Autodesk Inventor part; units mm, degrees
ref_plane "工作平面1" through (0, 5, 0) normal (0, -1, 0) x (1, 0, 0)
ref_plane "YZ Plane" through (0, 0, 0) normal (1, 0, 0) x (0, 1, 0)
ref_plane "XZ Plane" through (0, 0, 0) normal (0, 1, 0) x (-1, 0, 0)
sketch "草圖1" plane through (0, 0, 0) normal (0, 1, 0) x (-1, 0, 0)
  circle A0 centre (0, 0) radius 2.45
  dimension "d0" = 4.9
extrude "擠出1" add sketch "草圖1" along normal blind 160
ref_plane "工作平面1" through (0, 5, 0) normal (0, -1, 0) x (1, 0, 0)
sketch "草圖3" plane through (0, 5, 0) normal (0, -1, 0) x (1, 0, 0)
  circle A0 centre (0, 0) radius 2.45
  circle A1 centre (0, 0) radius 3.25
  line L0 (3.25, 0) -> (-3.25, 0)
  line L1 (-3.25, 0) -> (-3.25, -12)
  line L2 (-3.25, -12) -> (3.25, -12)
  line L3 (3.25, -12) -> (3.25, 0)
  line L4 (1.6, -12) -> (-1.6, -12)
  line L5 (-1.6, -12) -> (-1.6, -7)
  line L6 (-1.6, -7) -> (1.6, -7)
  line L7 (1.6, -7) -> (1.6, -12)
  line L8 (1.55, -7) -> (-1.55, -7)
  line L9 (-1.55, -7) -> (-1.55, -10.1)
  line L10 (-1.55, -10.1) -> (1.55, -10.1)
  line L11 (1.55, -10.1) -> (1.55, -7)
  line L12 (1.55, -10.1) -> (1.35, -10.1)
  line L13 (1.35, -10.1) -> (1.6, -12)
  line L14 (-1.55, -10.1) -> (-1.35, -10.1)
  line L15 (-1.35, -10.1) -> (-1.6, -12)
  circle A2 centre (0, -8.55) radius 2.192
  line L16 (-3.25, 0) -> (-3.25, 12)
  line L17 (-3.25, 12) -> (3.25, 12)
  line L18 (3.25, 12) -> (3.25, 0)
  line L19 (1.6, 12) -> (-1.6, 12)
  line L20 (-1.6, 12) -> (-1.6, 7)
  line L21 (-1.6, 7) -> (1.6, 7)
  line L22 (1.6, 7) -> (1.6, 12)
  line L23 (1.55, 7) -> (-1.55, 7)
  line L24 (-1.55, 7) -> (-1.55, 10.1)
  line L25 (-1.55, 10.1) -> (1.55, 10.1)
  line L26 (1.55, 10.1) -> (1.55, 7)
  line L27 (1.55, 10.1) -> (1.35, 10.1)
  line L28 (1.35, 10.1) -> (1.6, 12)
  line L29 (-1.55, 10.1) -> (-1.35, 10.1)
  line L30 (-1.35, 10.1) -> (-1.6, 12)
  circle A3 centre (0, 8.55) radius 2.192
  point P0 (0, -12)
  point P1 (0, -12)
  point P2 (0, -7)
  point P3 (-1.55, -7)
  point P4 (1.55, -7)
  point P5 (-1.55, -8.55)
  point P6 (-1.3711, -10.2603)
  point P7 (1.3711, -10.2603)
  point P8 (0, 12)
  point P9 (0, 12)
  point P10 (0, 7)
  point P11 (-1.55, 8.55)
  point P12 (1.3711, 10.2603)
  point P13 (-1.3711, 10.2603)
  point P14 (0.9915, 3.095)
  point P15 (-0.9915, 3.095)
  point P16 (-1.55, 10.1)
  point P17 (-1.55, -10.1)
  point P18 (-1.55, -10.1)
  dimension "d17" = 6.5
  dimension "d9" = 12
  dimension "d11" = 5
  dimension "d12" = 3.2
  dimension "d13" = 3.1
  dimension "d14" = 3.1
  dimension "d15" = 0.2
  dimension "d16" = 0.2
  dimension "d18" = 6.5
extrude "擠出3" add sketch "草圖3" against normal blind 3 contours L0 A1 A0 | A0 L0 A1 | L3 L2 L7 A2 L6 L5 L1 A1 | A1 L16 L17 L20 A3 L21 L22 L18 | L13 A2 L7 | L22 A3 L28 | L5 A2 L15 | L30 A3 L20 | L13 L10 A2 | A3 L25 L28 | A2 L10 L15 | L30 L25 A3 | A2 L6 L7 | L22 L21 A3 | L5 L6 A2 | A3 L21 L20
pattern_linear "矩形陣列1" count 6 spacing 30 along (0, 1, 0) of "擠出3"
properties part number "[3DP]double_bar"
Design review of the part built by this model. Coordinates are the model's own, in mm. A direction names the side the tool comes from. Round coordinates to 2 decimals unless told otherwise and drop trailing zeros. Order: outer loops, then holes, each group sorted by start corner. A loop starts at its lowest first (then second) coordinate and runs counter-clockwise, first axis right, second up.
1) Clearance check with flat-ended pins moving along their axes: pin 1 Ø2 at (x, z) = (-0.5, -1) entering from -Y; pin 2 Ø1 at (x, y) = (0, 91.5) entering from +Z; pin 3 Ø2 at (x, z) = (1, -5.5) entering from -Y; pin 4 Ø2 at (y, z) = (44.5, 1.5) entering from -X. State where each tip first meets the part, or that it passes through.
The answers:
pin 1: stops at y = 0
pin 2: stops at z = 2.45
pin 3: stops at y = 5
pin 4: stops at x = -2.4
2) Machinability: for faces 5 (the flat face through (-3.25, 156, 0)), 6 (the cylindrical face through (0.5, 159, 2.4)), which of the approach directions +Z, -Z, +X, -X, +Y, -Y give a long, thin tool a straight path to every point of the face, cutting with its end or side? Answer none if there is none.
The answers:
face 5: +Z, -Z, -X, +Y, -Y
face 6: +Y
3) Draft analysis for pull direction Z (two halves, no side actions). For faces 1 (the cylindrical face through (0.07, 36.48, -6.36)), 2 (the cylindrical face through (0.5, 141.3, 2.4)), 3 (the flat face through (3.25, 6, 0)), 4 (the cylindrical face through (0.07, 66.48, -6.36)), state which applies: released by +Z, released by -Z, zero draft, split by the parting line, or undercut.
The answers:
face 1: undercut
face 2: split by the parting line
face 3: zero draft
face 4: undercut
4) For L1, parallel to Y at x = 0.25, z = 4; L2, parallel to X at y = 67.1, z = -8.55; L3, parallel to Z at x = 0, y = 156.2, list the stretches that pass through material, from the lowest coordinate up.
The answers:
L1: y = 5 to 8, 35 to 38, 65 to 68, 95 to 98, 125 to 128, 155 to 158
L2: x = -3.25 to -2.19, 2.19 to 3.25
L3: z = -6.36 to 6.36
5) Consider section B-B (y = 75). State the section outline as (x, z) points.
The answers:
outline: circle Ø4.9 at (0, 0)
6) Consider section A-A (z = 4). State the section outline as (x, y) points, plus the area to 3 significant figures.
The answers:
outline: (-3.25, 5) - (3.25, 5) - (3.25, 8) - (-3.25, 8) - close; (-3.25, 35) - (3.25, 35) - (3.25, 38) - (-3.25, 38) - close; (-3.25, 65) - (3.25, 65) - (3.25, 68) - (-3.25, 68) - close; (-3.25, 95) - (3.25, 95) - (3.25, 98) - (-3.25, 98) - close; (-3.25, 125) - (3.25, 125) - (3.25, 128) - (-3.25, 128) - close; (-3.25, 155) - (3.25, 155) - (3.25, 158) - (-3.25, 158) - close
area: 117 mm2
7) Consider section C-C (z = -8.55). Count the separate pieces of the cut face and the enclosed holes in it, plus the area to 3 significant figures.
The answers:
separate pieces: 12
enclosed holes: 0
area: 38.1 mm2
